from build123d import *

# Parameters (mm, degrees)
F0_W     = 150
F0_H     = 150
F1_DEPTH = 50
F2_W     = 130
F2_H     = 130
F3_DEPTH = 35
F4_W     = 40
F4_H     = 10
F5_DEPTH = 150.001


with BuildPart() as f1:
    # F0 (on Top) → F1 (new body)
    with BuildSketch(Plane.XY):
        Rectangle(F0_W, F0_H)
    extrude(amount=F1_DEPTH)

    # F2 (on face) → F3 (cut)
    with BuildSketch(Plane.XY.offset(50)):
        Rectangle(F2_W, F2_H)
    extrude(amount=-F3_DEPTH, mode=Mode.SUBTRACT)

    # F4 (on face) → F5 (cut, through all)
    with BuildSketch(Plane.YZ.offset(75)):
        with Locations((0, 35)):
            Rectangle(F4_W, F4_H)
    extrude(amount=-F5_DEPTH, mode=Mode.SUBTRACT)


solid = f1.part
The listing builds one solid part. Answer for the finished solid, in the listing's coordinates (mm). A direction names the side the tool comes from. Round coordinates to 2 decimals unless told otherwise and drop trailing zeros. Write each loop counter-clockwise with the first axis right and the second up, starting at its lowest first coordinate (ties: lowest second). Pieces come first, ordered by that corner, then holes. Notation, with made-up numbers: M 9,-11 L 64,-11 A9 ccw 64,-6 Z; hole C 68.5,83.25 d1. An arc over 180 degrees is marked long. Write each question's results on one line, items separated by ' | '. Start each with the question number.
Item 1: For a pull along Y with two mould halves and no side action, classify faces 4 (the face through (-1, -75, 25)), 5 (the face through (-70, 0, 40)), 6 (the face through (75, -1, 25)), 7 (the face through (-65, -1, 29)) as pulls with the +Y half, pulls with the -Y half, needs draft (parallel to the pull), parting line crosses it, or undercut.
Item 2: A cutting plane is placed at B-B on z = 36.5. Write down the section's boundary in (x, y), and give its area (3 significant figures).
Item 3: A cutting plane is placed at A-A on y = 9.5. Write down the section's boundary in (x, z).
Item 4: A cutting plane is placed at D-D on y = -55.5. Write down the section's boundary in (x, z).
Item 5: Straight lines are drawn through the part: L1, parallel to Y at x = 62, z = 38.5; L2, parallel to Z at x = -27, y = -39. For each, find the intervals that lie inside material, in ascending order. Write a range as [from, to].
Item 6: For faces 1 (the face through (-70, 0, 30)), 2 (the face through (-1, 65, 33)), 3 (the face through (-1, 1, 0)), determine the directions among +Z, -Z, +X, -X, +Y, -Y from which every point of the face is accessible in a straight line to the end or side of a thin tool.
Item 7: A cutting plane is placed at C-C on z = 27. Write down the section's boundary in (x, y), and give its area (3 significant figures).
Item 8: A flat-ended cylindrical pin translates along its axis: pin 1 Ø2 at (x, y) = (39, 29) entering from +Z. Find the tip coordinate at first contact, or state that the pin passes through.
Check sheet entries:
1) face 4: pulls with the -Y half | face 5: undercut | face 6: needs draft | face 7: undercut
2) outline: M -75,-75 L 75,-75 L 75,-20 L 65,-20 L 65,-65 L -65,-65 L -65,-20 L -75,-20 Z; M -75,20 L -65,20 L -65,65 L 65,65 L 65,20 L 75,20 L 75,75 L -75,75 Z | area: 4,800 mm²
3) outline: M -75,0 L 75,0 L 75,30 L 65,30 L 65,15 L -65,15 L -65,30 L -75,30 Z; M -75,40 L -65,40 L -65,50 L -75,50 Z; M 65,40 L 75,40 L 75,50 L 65,50 Z
4) outline: M -75,0 L 75,0 L 75,50 L 65,50 L 65,15 L -65,15 L -65,50 L -75,50 Z
5) L1: [-75, -65], [65, 75] | L2: [0, 15]
6) face 1: +X, -X | face 2: +Z | face 3: -Z, +X, -X, +Y, -Y
7) outline: M -75,-75 L 75,-75 L 75,75 L -75,75 Z; hole M -65,-65 L 65,-65 L 65,65 L -65,65 Z | area: 5,600 mm²
8) pin 1: z = 15
